For this review, take the finished solid that the model builds, in its own axes (mm). Face numbers are marked on the shaded views. A direction names the side the tool comes from. Coordinates: 2 decimals unless noted, no trailing zeros. Loops run counter-clockwise (first coordinate to the right, second up) from the corner with the lowest first, then second, coordinate; pieces in that order, holes last. Notation, with made-up numbers: M 5,3.5 L 16,3.5 A12 cw 16,25.5 Z; hole C 47,37 d3. An arc over 180 degrees is marked long. Write item = value, one per line.
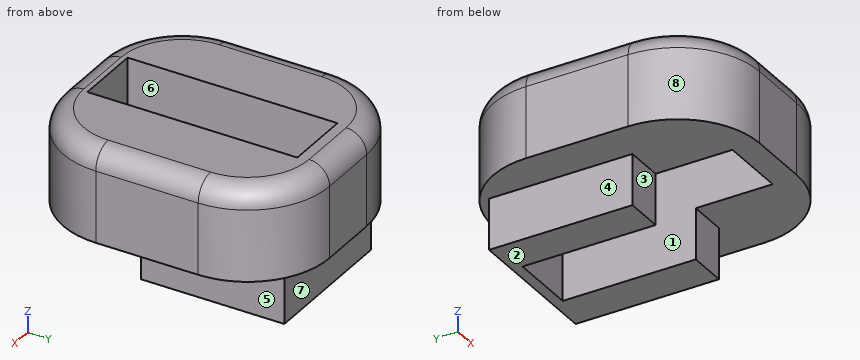
from build123d import *

# Parameters (mm, degrees)
F0_W     = 14
F0_H     = 14
F1_DEPTH = 5
F2_W     = 22
F2_H     = 26
F2_W_2   = 14
F2_H_2   = 14
F3_DEPTH = 9
F4_W     = 6.5
F4_H     = 20.5
F5_DEPTH = 9
F6_W     = 6.5
F6_H     = 13
F7_DEPTH = 5.001
F8_R     = 8
F9_R     = 2


with BuildPart() as f1:
    # F0 (on Top) → F1 (new body)
    with BuildSketch(Plane.XY):
        with Locations((-7, 7)):
            Rectangle(F0_W, F0_H)
    extrude(amount=F1_DEPTH)

    # F2 (on face) → F3 (join)
    with BuildSketch(Plane.XY.offset(5)):
        with Locations((-7, 3)):
            Rectangle(F2_W, F2_H)
        with Locations((-7, 7)):
            Rectangle(F2_W_2, F2_H_2, mode=Mode.SUBTRACT)
        with Locations((-7, 7)):
            Rectangle(F2_W_2, F2_H_2)
    extrude(amount=F3_DEPTH)

    # F4 (on face) → F5 (cut, through all)
    with BuildSketch(Plane.XY.offset(14)):
        with Locations((-7, 2.75)):
            Rectangle(F4_W, F4_H)
    extrude(amount=-F5_DEPTH, mode=Mode.SUBTRACT)

    # F6 (on face) → F7 (cut, through all)
    with BuildSketch(Plane.XY.offset(5)):
        with Locations((-7, 6.5)):
            Rectangle(F6_W, F6_H)
    extrude(amount=-F7_DEPTH, mode=Mode.SUBTRACT)

    # F8
    f8_edges = [f1.edges().sort_by_distance(p)[0] for p in [
        (4, -10, 9.5),
        (4, 16, 9.5),
        (-18, 16, 9.5),
        (-18, -10, 9.5),
    ]]
    fillet(f8_edges, radius=F8_R)

    # F9
    f9_edges = [f1.edges().sort_by_distance(p)[0] for p in [
        (4, 3, 14),
        (1.656854, 13.656854, 14),
    ]]
    fillet(f9_edges, radius=F9_R)


solid = f1.part
Q1. Draft analysis for pull direction Y (two halves, no side actions). For the marked faces 6, 7 and 8, state which applies: +Y half, -Y half, draft (parallel to the pull), parting line (faces both ways), or undercut.
Solved:
face_6 = undercut
face_7 = +Y half
face_8 = -Y half
Q2. For pin 1 Ø4 at (x, z) = (-12, 1.5) entering from -Y; pin 2 Ø1 at (x, z) = (-12.5, 6.5) entering from +Y; pin 3 Ø1.5 at (y, z) = (9, 3) entering from -X, all flat-tipped, find the tip position at first contact; note any pin that passes through.
Solved:
pin_1 = 0
pin_2 = 15.75
pin_3 = -14
Q3. Machinability: for the marked faces 1, 2, 3, 4 and 5, which of the approach directions +Z, -Z, +X, -X, +Y, -Y give a long, thin tool a straight path to every point of the face, cutting with its end or side? Answer none if there is none.
Solved:
face_1 = +Z, -Z
face_2 = -Z, +X, -X, +Y, -Y
face_3 = -Z, +X, -X, -Y
face_4 = -Z, -X, +Y, -Y
face_5 = -Z, +X, +Y, -Y
Q4. Add section C-C (x = -7.25). Write out the cut boundary in (y, z), and give its area (3 significant figures).
Solved:
outline = M -10,5 L -7.5,5 L -7.5,14 L -8,14 A2 ccw -10,12 Z; M 13,0 L 14,0 L 14,5 L 16,5 L 16,12 A2 ccw 14,14 L 13,14 Z
area = 52.8 mm²
Q5. Add section A-A (y = -1). Write out the cut boundary in (x, z).
Solved:
outline = M -18,5 L -10.25,5 L -10.25,14 L -16,14 A2 ccw -18,12 Z; M -3.75,5 L 4,5 L 4,12 A2 ccw 2,14 L -3.75,14 Z
Q6. Add section B-B (z = 6.5). Write out the cut boundary in (x, y).
Solved:
outline = M -18,-2 A8 ccw -10,-10 L -4,-10 A8 ccw 4,-2 L 4,8 A8 ccw -4,16 L -10,16 A8 ccw -18,8 Z; hole M -10.25,-7.5 L -3.75,-7.5 L -3.75,13 L -10.25,13 Z
Q7. For line 1 along Y through (x, z) = (-7.25, 8); line 2 along X through (y, z) = (1.5, 7.5); line 3 along X through (y, z) = (1.75, 4), list the stretches that pass through material, from the lowest coordinate up.
Solved:
line_1 = -10 to -7.5, 13 to 16
line_2 = -18 to -10.25, -3.75 to 4
line_3 = -14 to -10.25, -3.75 to 0
Q8. Add section D-D (z = 4). Write out the cut boundary in (x, y), and give its area (4 significant figures).
Solved:
outline = M -14,0 L -10.25,0 L -10.25,13 L -3.75,13 L -3.75,0 L 0,0 L 0,14 L -14,14 Z
area = 111.5 mm²
